For this review, take the finished solid that the model builds, in its own axes (mm). Face numbers are marked on the shaded views. A direction names the side the tool comes from. Coordinates: 2 decimals unless noted, no trailing zeros. Write each loop counter-clockwise with the first axis right and the second up, starting at its lowest first coordinate (ties: lowest second). Pieces come first, ordered by that corner, then holes. Notation, with made-up numbers: (29, 21.5) - (71, 21.5) arc R23 ccw to (71, 40.5) - close; hole circle Ø7 at (5.25, -13). An arc over 180 degrees is marked (long way). Write each question's results on one line, items separated by ' | '.
from build123d import *

# Parameters (mm, degrees)
F1_DEPTH = 31.75
F3_DEPTH = 25.732862
F5_DEPTH = 12.7
F7_DEPTH = 12.7


with BuildPart() as f1:
    # F0 (on Front) → F1 (new body)
    with BuildSketch(Plane.XZ):
        Polygon((-17.791169, 49.352903), (-56.388959, 49.352903), (-56.388959, 17.590139), (-43.523028, 17.590139), (-43.523028, -7.940691), (-30.657098, -7.940691), (-30.657098, 17.590139), (-17.791169, 17.590139), align=None)
    extrude(amount=F1_DEPTH)

    # F2 (on face) → F3 (cut, through all)
    with BuildSketch(Plane.YZ.offset(-30.657098)):
        Polygon((0, -7.940691), (-31.75, 4.759309), (-31.75, -7.940691), align=None)
    extrude(amount=-F3_DEPTH, mode=Mode.SUBTRACT)

    # F4 (on face) → F5 (cut)
    with BuildSketch(Plane(origin=(-56.388959, 0, 0), x_dir=(0, -1, 0), z_dir=(-1, 0, 0))):
        Polygon((31.75, 17.590139), (31.75, 30.290139), (0, 17.590139), align=None)
    extrude(amount=-F5_DEPTH, mode=Mode.SUBTRACT)

    # F6 (on face) → F7 (cut)
    with BuildSketch(Plane.YZ.offset(-17.791169)):
        Polygon((0, 17.590139), (-31.75, 30.290139), (-31.75, 17.590139), align=None)
    extrude(amount=-F7_DEPTH, mode=Mode.SUBTRACT)


solid = f1.part
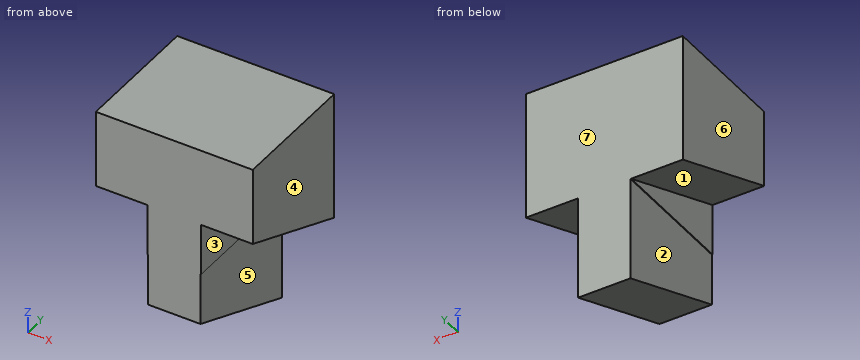
Q1. Take a section at A-A on z = 25. State the section outline as (x, y) points.
Results found:
outline: (-56.39, -18.52) - (-43.69, -18.52) - (-43.69, -31.75) - (-30.49, -31.75) - (-30.49, -18.52) - (-17.79, -18.52) - (-17.79, 0) - (-56.39, 0) - close
Q2. Wall thickness on line 1 along X through (y, z) = (-24, 4.5); line 2 along Z through (x, y) = (-22.5, -22); line 3 along Z through (x, y) = (-51, -5): over which ranges is each line inside the solid? List them lowest first. Write a range as from..to.
Results found:
line 1: -43.52..-30.66 | line 2: 26.39..49.35 | line 3: 19.59..49.35
Q3. Take a section at D-D on y = -10. State the section outline as (x, z) points, plus the area to 3 significant figures.
Results found:
outline: (-56.39, 21.59) - (-43.69, 21.59) - (-43.69, 17.59) - (-43.52, 17.59) - (-43.52, -3.94) - (-30.66, -3.94) - (-30.66, 17.59) - (-30.49, 17.59) - (-30.49, 21.59) - (-17.79, 21.59) - (-17.79, 49.35) - (-56.39, 49.35) - close | area: 1,400 mm2
Q4. Take a section at C-C on y = -20. State the section outline as (x, z) points.
Results found:
outline: (-56.39, 25.59) - (-43.69, 25.59) - (-43.69, 17.59) - (-43.52, 17.59) - (-43.52, 0.06) - (-30.66, 0.06) - (-30.66, 17.59) - (-30.49, 17.59) - (-30.49, 25.59) - (-17.79, 25.59) - (-17.79, 49.35) - (-56.39, 49.35) - close
Q5. For pin 1 (5 mm diameter, centred on y = -10, z = 5, fed in from -X); pin 2 (6 mm diameter, centred on y = -9, z = 16.5, fed in from +X); pin 3 (10 mm diameter, centred on x = -26.5, y = -22, fed in from -Z), all flat-tipped, find the tip position at first contact; note any pin that passes through.
Results found:
pin 1: x = -43.52 | pin 2: x = -30.49 | pin 3: z = -0.25
Q6. Take a section at B-B on x = -19.5. State the section outline as (y, z) points.
Results found:
outline: (-31.75, 30.29) - (0, 17.59) - (0, 49.35) - (-31.75, 49.35) - close
Q7. For the marked faces 1, 2, 3 and 4, list the 3-axis set-ups (+Z, -Z, +X, -X, +Y, -Y) from which the entire face can be reached by the end or side of a thin tool; tool diameter is ignored.
Results found:
face 1: -Z, -X, -Y | face 2: -Z, -X, +Y, -Y | face 3: -Z, +X, -Y | face 4: +Z, -Z, +X, +Y, -Y
Q8. Mouldability with a two-part tool opening along X and no side actions: class the marked faces 5, 6 and 7 as pulls with the +X half, pulls with the -X half, needs draft (parallel to the pull), parting line crosses it, or undercut.
Results found:
face 5: pulls with the +X half | face 6: pulls with the -X half | face 7: needs draft
